```python
from build123d import *

# Parameters (mm, degrees)
SKETCH1_W           = 75
SKETCH1_H           = 63
BOSS_EXTRUDE1_DEPTH = 12
SKETCH2_W           = 25
SKETCH2_H           = 25
BOSS_EXTRUDE2_DEPTH = 63
CUT_EXTRUDE1_DEPTH  = 114
BOSS_EXTRUDE3_DEPTH = 63
SKETCH6_W           = 25
SKETCH6_H           = 12
CUT_EXTRUDE2_DEPTH  = 15
BOSS_EXTRUDE5_DEPTH = 48
SKETCH8_W           = 12
SKETCH8_H           = 19
CUT_EXTRUDE3_DEPTH  = 25
SKETCH9_W           = 25
SKETCH9_H           = 25
BOSS_EXTRUDE7_DEPTH = 44
CUT_EXTRUDE7_DEPTH  = 44
CUT_EXTRUDE8_DEPTH  = 44


with BuildPart() as part:
    # Sketch1 → Boss-Extrude1 (new body)
    with BuildSketch(Plane.XY):
        with Locations((37.5, -31.5)):
            Rectangle(SKETCH1_W, SKETCH1_H)
    extrude(amount=BOSS_EXTRUDE1_DEPTH)

    # Sketch2 → Boss-Extrude2 (add)
    with BuildSketch(Plane(origin=(0, -63, 0), x_dir=(-1, 0, 0), z_dir=(0, -1, 0))):
        with Locations((-12.5, -12.5)):
            Rectangle(SKETCH2_W, SKETCH2_H)
    extrude(amount=-BOSS_EXTRUDE2_DEPTH)

    # Sketch3 → Cut-Extrude1 (cut)
    with BuildSketch(Plane(origin=(0, -63, 0), x_dir=(-1, 0, 0), z_dir=(0, -1, 0))):
        Polygon((-25, -25), (0, -12), (0, -25), align=None)
    extrude(amount=-CUT_EXTRUDE1_DEPTH, mode=Mode.SUBTRACT)

    # Sketch4 → Boss-Extrude3 (add)
    with BuildSketch(Plane.XZ.offset(63)):
        Polygon((75, 50), (50, 38), (50, 0), (75, 0), align=None)
    extrude(amount=-BOSS_EXTRUDE3_DEPTH)

    # Sketch6 → Cut-Extrude2 (cut)
    with BuildSketch(Plane.XZ.offset(63)):
        with Locations((37.5, 6)):
            Rectangle(SKETCH6_W, SKETCH6_H)
    extrude(amount=-CUT_EXTRUDE2_DEPTH, mode=Mode.SUBTRACT)

    # Sketch7 → Boss-Extrude5 (add)
    with BuildSketch(Plane.XZ.offset(48)):
        Polygon((50, 38), (50, 12), (25, 12), (25, 25), align=None)
    extrude(amount=-BOSS_EXTRUDE5_DEPTH)

    # Sketch8 → Cut-Extrude3 (cut)
    with BuildSketch(Plane(origin=(75, 0, 0), x_dir=(0, 0, -1), z_dir=(1, 0, 0))):
        with Locations((-44, -31.5)):
            Rectangle(SKETCH8_W, SKETCH8_H)
    extrude(amount=-CUT_EXTRUDE3_DEPTH, mode=Mode.SUBTRACT)

    # Sketch9 → Boss-Extrude7 (add)
    with BuildSketch(Plane(origin=(-4.911838791, 0, 9.445843829), x_dir=(0.887216801234595, 0, 0.4613527366419899), z_dir=(-0.4613527366419899, 0, 0.887216801234595))):
        with Locations((30.03623284, -31.5)):
            Rectangle(SKETCH9_W, SKETCH9_H)
    extrude(amount=BOSS_EXTRUDE7_DEPTH)

    # Sketch12 → Cut-Extrude7 (cut)
    with BuildSketch(Plane(origin=(0, -44, 0), x_dir=(-1, 0, 0), z_dir=(0, -1, 0))):
        Polygon((-3.264957829, -31.731701659), (9.652918797, -56.573772094), (-12.527501233, -68.10759051), (-32.827021646, -29.070051256), align=None)
    extrude(amount=-CUT_EXTRUDE7_DEPTH, mode=Mode.SUBTRACT)

    # Sketch13 → Cut-Extrude8 (cut)
    with BuildSketch(Plane.XZ.offset(44)):
        Polygon((32.827021646, 29.070051256), (5.896218628, 26.671584738), (3.264957829, 31.731701659), align=None)
    extrude(amount=-CUT_EXTRUDE8_DEPTH, mode=Mode.SUBTRACT)


solid = part.part
```
Build history of the part. All positions in model axes, mm. A direction names the side the tool comes from. Round coordinates to 2 decimals unless told otherwise and drop trailing zeros. Order: outer loops, then holes, each group sorted by start corner. A loop starts at its lowest first (then second) coordinate and runs counter-clockwise, first axis right, second up. Notation, with made-up numbers: (88, -6.75) -> (98, -6.75) arc R9 ccw to (98, 9.25) -> close; hole circle Ø1 at (-13.75, 19). An arc over 180 degrees is marked (long way). Answer in a Markdown table with one row per item.
1) Pin check, flat tips, straight feed: P1, Ø10, axis at x = 49, y = -15, coming from the +Z side; P2, Ø2, axis at y = -22, z = 41, coming from the -X side; P3, Ø7.5, axis at x = 34.5, z = 13.5, coming from the -Y side. Stop position of each tip, or through.
Values:
| item | result |
|---|---|
| P1 | z = 39.92 |
| P2 | x = 54.17 |
| P3 | y = -48 |
2) Wall check: L1, parallel to X at y = -52, z = 10; L2, parallel to Y at x = 28, z = 11; L3, parallel to Z at x = 53, y = -29.5. Give the ranges that are in metal, low to high.
Values:
| item | result |
|---|---|
| L1 | 0 to 25, 50 to 75 |
| L2 | -48 to 0 |
| L3 | 0 to 38 |
3) Band-saw the part on D-D on y = -46. Give the cut face in (x, z), and give its area (3 significant figures).
Values:
| item | result |
|---|---|
| outline | (0, 0) -> (75, 0) -> (75, 50) -> (50, 38) -> (0, 12) -> close |
| area | 2,350 mm2 |
4) Band-saw the part on B-B on z = 5. Give the cut face in (x, y).
Values:
| item | result |
|---|---|
| outline | (0, -63) -> (25, -63) -> (25, -48) -> (50, -48) -> (50, -63) -> (75, -63) -> (75, 0) -> (0, 0) -> close |
5) Band-saw the part on A-A on y = -58. Give the cut face in (x, z), and give its area (3 significant figures).
Values:
| item | result |
|---|---|
| outline | (0, 0) -> (25, 0) -> (25, 25) -> (0, 12) -> close; (50, 0) -> (75, 0) -> (75, 50) -> (50, 38) -> close |
| area | 1,560 mm2 |
6) Which spindle directions (+Z, -Z, +X, -X, +Y, -Y) get a long thin tool onto all of the face, cutting with end or side? Do faces 4 (the flat face through (8.305, -31.675, 22.04)), 5 (the flat face through (25, -56, 13)), 6 (the flat face through (68, -41, 41)). Say none if no direction does.
Values:
| item | result |
|---|---|
| face 4 | -X, +Y, -Y |
| face 5 | +Z, -Z, -Y |
| face 6 | +Z, +X, -X |
7) Mould opens along X. For faces 1 (the flat face through (50, -56, 19)), 2 (the flat face through (68, -22, 41)), 3 (the flat face through (25, -18, 25)) say: released by +X, released by -X, zero draft, split by the parting line, or undercut.
Values:
| item | result |
|---|---|
| face 1 | undercut |
| face 2 | zero draft |
| face 3 | released by -X |
8) Band-saw the part on C-C on x = 60. Give the cut face in (y, z), and give its area (3 significant figures).
Values:
| item | result |
|---|---|
| outline | (-63, 0) -> (0, 0) -> (0, 42.8) -> (-22, 42.8) -> (-22, 38) -> (-41, 38) -> (-41, 42.8) -> (-63, 42.8) -> close |
| area | 2,610 mm2 |
